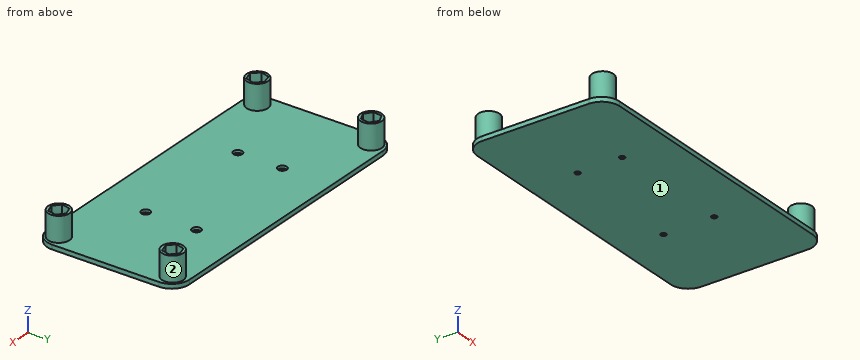
from build123d import *

# Parameters (mm, degrees)
EXTRUDE_1_DEPTH          = 2.5
CUT_EXTRUDE_1_DEPTH      = 42
CUT_EXTRUDE_1_DEPTH_BACK = 10
SKETCH_2_R               = 1.5
SKETCH_3_R               = 2.5
CUT_EXTRUDE_2_DEPTH      = 1.5
SKETCH_7_R               = 6
EXTRUDE_4_DEPTH          = 14
BUTTON_LEFT_NUT_DEPTH    = 5
UP_LEFT_NUT_DEPTH        = 5
UP_RIGHT_NUT_DEPTH       = 5
BUTTON_RIGHT_NUT_DEPTH   = 5
SKETCH_13_R              = 3.25
CUT_EXTRUDE_7_DEPTH      = 13
SKETCH_15_R              = 3.25
CUT_EXTRUDE_8_DEPTH      = 13
SKETCH_16_R              = 3.25
CUT_EXTRUDE_9_DEPTH      = 13
SKETCH_17_R              = 3.25
CUT_EXTRUDE_10_DEPTH     = 13


with BuildPart() as part:
    # 草图1 → 凸台-拉伸1 (new body)
    with BuildSketch(Plane.XY):
        with BuildLine():
            Line((-72.574116531, 35.487390308), (77.425883469, 35.487390308))
            ThreePointArc((77.425883469, 35.487390308), (84.496951281, 32.558458119), (87.425883469, 25.487390308))
            Line((87.425883469, 25.487390308), (87.425883469, -34.512609692))
            ThreePointArc((87.425883469, -34.512609692), (84.496951281, -41.583677504), (77.425883469, -44.512609692))
            Line((77.425883469, -44.512609692), (-72.574116531, -44.512609692))
            ThreePointArc((-72.574116531, -44.512609692), (-79.645184343, -41.583677504), (-82.574116531, -34.512609692))
            Line((-82.574116531, -34.512609692), (-82.574116531, 25.487390308))
            ThreePointArc((-82.574116531, 25.487390308), (-79.645184343, 32.558458119), (-72.574116531, 35.487390308))
        make_face()
    extrude(amount=EXTRUDE_1_DEPTH)

    # 草图2 → 切除-拉伸1 (cut, two sides: drawn at the far end of the back side and taken through both)
    with BuildSketch(Plane.XY.offset(2.5).offset(-CUT_EXTRUDE_1_DEPTH_BACK)):
        with Locations((-32.574116531, 7.987390308)):
            Circle(SKETCH_2_R)
        with Locations((-32.574116531, -17.012609692)):
            Circle(SKETCH_2_R)
        with Locations((37.425883469, 10.450230815)):
            Circle(SKETCH_2_R)
        with Locations((37.425883469, -18.090102414)):
            Circle(SKETCH_2_R)
    extrude(amount=CUT_EXTRUDE_1_DEPTH + CUT_EXTRUDE_1_DEPTH_BACK, mode=Mode.SUBTRACT)

    # 草图3 → 切除-拉伸2 (cut)
    with BuildSketch(Plane.XY.offset(2.5)):
        with Locations((-32.574116531, 7.987390308)):
            Circle(SKETCH_3_R)
        with Locations((37.425883469, 10.450230815)):
            Circle(SKETCH_3_R)
        with Locations((37.425883469, -18.090102414)):
            Circle(SKETCH_3_R)
        with Locations((-32.574116531, -17.012609692)):
            Circle(SKETCH_3_R)
    extrude(amount=-CUT_EXTRUDE_2_DEPTH, mode=Mode.SUBTRACT)

    # 草图7 → 凸台-拉伸4 (add)
    with BuildSketch(Plane.XY.offset(2.5)):
        with Locations(Location((-74.574116531, 27.487390308, 0), (0, 0, 180))):
            Circle(SKETCH_7_R)
        with Locations(Location((-74.574116531, -36.512609692, 0), (0, 0, 180))):
            Circle(SKETCH_7_R)
        with Locations(Location((79.425883469, 27.487390308, 0), (0, 0, 180))):
            Circle(SKETCH_7_R)
        with Locations(Location((79.425883469, -36.512609692, 0), (0, 0, 180))):
            Circle(SKETCH_7_R)
    extrude(amount=EXTRUDE_4_DEPTH)

    # 草图9 → button left nut (cut)
    with BuildSketch(Plane.XY.offset(16.5)):
        Polygon((-70.944636645, -40.226166125), (-69.543342379, -35.226166125), (-73.172822265, -31.512609692), (-78.203596417, -32.79905326), (-79.604890683, -37.79905326), (-75.975410797, -41.512609692), align=None)
    extrude(amount=-BUTTON_LEFT_NUT_DEPTH, mode=Mode.SUBTRACT)

    # 草图10 → up left nut (cut)
    with BuildSketch(Plane.XY.offset(16.5)):
        Polygon((-70.484611493, 24.610595469), (-70.0379866, 29.59060814), (-74.127491638, 32.467402979), (-78.663621569, 30.364185146), (-79.110246462, 25.384172475), (-75.020741423, 22.507377636), align=None)
    extrude(amount=-UP_LEFT_NUT_DEPTH, mode=Mode.SUBTRACT)

    # 草图11 → up right nut (cut)
    with BuildSketch(Plane.XY.offset(16.5)):
        Polygon((83.054173559, 24.047112554), (84.219396445, 28.909442821), (80.591106355, 32.349720575), (75.797593379, 30.927668061), (74.632370493, 26.065337794), (78.260660583, 22.62506004), align=None)
    extrude(amount=-UP_RIGHT_NUT_DEPTH, mode=Mode.SUBTRACT)

    # 草图12 → button right nut (cut)
    with BuildSketch(Plane.XY.offset(16.5)):
        Polygon((83.162930062, -39.834428887), (84.171186575, -34.937142005), (80.434139981, -31.61532281), (75.688836876, -33.190790498), (74.680580363, -38.08807738), (78.417626957, -41.409896575), align=None)
    extrude(amount=-BUTTON_RIGHT_NUT_DEPTH, mode=Mode.SUBTRACT)

    # 草图13 → 切除-拉伸7 (cut)
    with BuildSketch(Plane.XY.offset(16.5)):
        with Locations((-74.574116531, -36.512609692)):
            Circle(SKETCH_13_R)
    extrude(amount=-CUT_EXTRUDE_7_DEPTH, mode=Mode.SUBTRACT)

    # 草图15 → 切除-拉伸8 (cut)
    with BuildSketch(Plane.XY.offset(16.5)):
        with Locations((-74.574116531, 27.487390308)):
            Circle(SKETCH_15_R)
    extrude(amount=-CUT_EXTRUDE_8_DEPTH, mode=Mode.SUBTRACT)

    # 草图16 → 切除-拉伸9 (cut)
    with BuildSketch(Plane.XY.offset(16.5)):
        with Locations((79.425883469, 27.487390308)):
            Circle(SKETCH_16_R)
    extrude(amount=-CUT_EXTRUDE_9_DEPTH, mode=Mode.SUBTRACT)

    # 草图17 → 切除-拉伸10 (cut)
    with BuildSketch(Plane.XY.offset(16.5)):
        with Locations((79.425883469, -36.512609692)):
            Circle(SKETCH_17_R)
    extrude(amount=-CUT_EXTRUDE_10_DEPTH, mode=Mode.SUBTRACT)


solid = part.part
Work out the finished part from the listing and answer in its coordinate system (mm). Face numbers are marked on the shaded views. Give positions to 0.01 mm unless a question says otherwise; leave off trailing zeros. Loops run counter-clockwise (first coordinate to the right, second up) from the corner with the lowest first, then second, coordinate; pieces in that order, holes last. Notation, with made-up numbers: (41.25, -23.5) - (92.25, -23.5) arc R19 ccw to (92.25, 5.5) - close; hole circle Ø4 at (19, 48.25). An arc over 180 degrees is marked (long way). Answer in a Markdown table with one row per item.
(1) Flat-ended cylindrical pins translate along their axes: pin 1 Ø1.5 at (x, z) = (59, 5) entering from -Y; pin 2 Ø5.5 at (x, y) = (-33.5, 9) entering from +Z; pin 3 Ø5 at (x, y) = (-75.5, -36.5) entering from +Z; pin 4 Ø3.5 at (x, y) = (-32.57, -17.01) entering from +Z. Find the tip coordinate at first contact, or state that the pin passes through.
Results list:
| item | result |
|---|---|
| pin 1 | passes through |
| pin 2 | stops at z = 2.5 |
| pin 3 | stops at z = 11.5 |
| pin 4 | stops at z = 1 |
(2) Consider L1, parallel to Z at x = 14.5, y = 32.5; L2, parallel to X at y = -41, z = 3; L3, parallel to X at y = 22, z = 3.25. Determine where each line is inside the solid, lowest interval first. Write a range as [from, to].
Results list:
| item | result |
|---|---|
| L1 | z = [0, 2.5] |
| L2 | x = [-78.56, -70.59], [75.44, 83.41] |
| L3 | x = [-77, -72.15], [77, 81.85] |
(3) Section C-C (x = -54) is taken. Give the vertices of the cut face in (y, z), and give its area (3 significant figures).
Results list:
| item | result |
|---|---|
| outline | (-44.51, 0) - (35.49, 0) - (35.49, 2.5) - (-44.51, 2.5) - close |
| area | 200 mm² |
(4) Section B-B (y = 1.5) is taken. Give the vertices of the cut face in (x, z), and give its area (3 significant figures).
Results list:
| item | result |
|---|---|
| outline | (-82.57, 0) - (87.43, 0) - (87.43, 2.5) - (-82.57, 2.5) - close |
| area | 425 mm² |
(5) Section A-A (z = 7.5) is taken. Give the vertices of the cut face in (x, y), and give its area (3 significant figures).
Results list:
| item | result |
|---|---|
| outline | circle Ø12 at (-74.57, -36.51); circle Ø12 at (-74.57, 27.49); circle Ø12 at (79.43, -36.51); circle Ø12 at (79.43, 27.49); hole circle Ø6.5 at (-74.57, -36.51); hole circle Ø6.5 at (-74.57, 27.49); hole circle Ø6.5 at (79.43, -36.51); hole circle Ø6.5 at (79.43, 27.49) |
| area | 320 mm² |
(6) For a pull along Y with two mould halves and no side action, classify the marked faces 1 and 2 as pulls with the +Y half, pulls with the -Y half, needs draft (parallel to the pull), parting line crosses it, or undercut.
Results list:
| item | result |
|---|---|
| face 1 | needs draft |
| face 2 | undercut |
